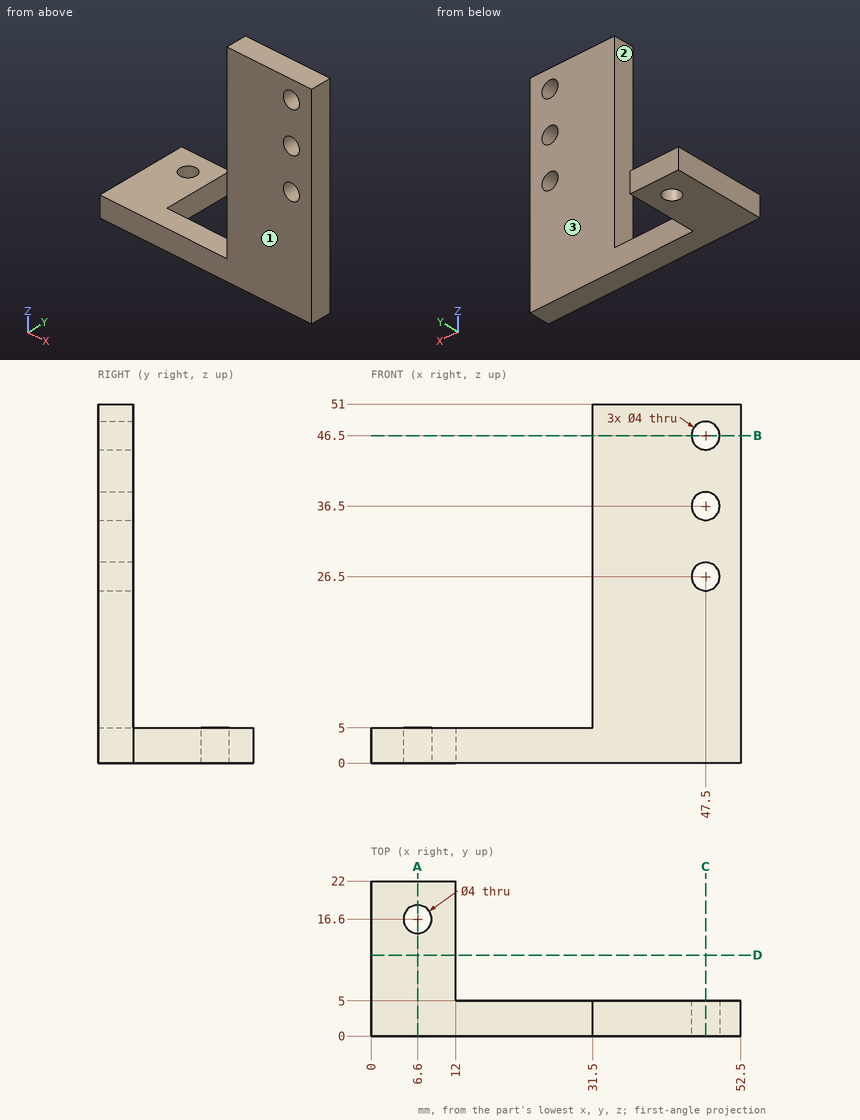
Design review of the part shown in the three views and the two pictorial views. Dimensions are in mm from the part's minimum x, y and z. A direction names the side the tool comes from. Give positions to 0.01 mm unless a question says otherwise; leave off trailing zeros. Loops run counter-clockwise (first coordinate to the right, second up) from the corner with the lowest first, then second, coordinate; pieces in that order, holes last. Notation, with made-up numbers: M -19,14 L 4,14 A19 ccw 4,50 Z; hole C 24,72 d7. An arc over 180 degrees is marked long. Put each result on its own line as item: value. Start each with the question number.
(1) Add section A-A, the plane x = 6.6. Write out the cut boundary in (y, z).
(2) Wall thickness on L1, parallel to X at y = 1.2, z = 46.5; L2, parallel to Y at x = 37.5, z = 25; L3, parallel to X at y = 2, z = 23: over which ranges is each line inside the solid? List them lowest first.
(3) Add section C-C, the plane x = 47.5. Write out the cut boundary in (y, z).
(4) Add section B-B, the plane z = 46.5. Write out the cut boundary in (x, y), then the cut area to 3 significant figures.
(5) Machinability: for the marked faces 1, 2 and 3, which of the approach directions +Z, -Z, +X, -X, +Y, -Y give a long, thin tool a straight path to every point of the face, cutting with its end or side? Answer none if there is none.
(6) For pin 1 (6.5 mm diameter, centred on x = 47.5, z = 36.5, fed in from +Y); pin 2 (2.5 mm diameter, centred on x = 6.6, y = 16.6, fed in from +Z); pin 3 (5.5 mm diameter, centred on y = 3, z = 32, fed in from -X); pin 4 (5.5 mm diameter, centred on y = 12, z = 3, fed in from +X), all flat-tipped, find the tip position at first contact; note any pin that passes through.
(7) Add section D-D, the plane y = 11.5. Write out the cut boundary in (x, z).
Result:
1. outline: M 0,0 L 14.6,0 L 14.6,5 L 0,5 Z; M 18.6,0 L 22,0 L 22,5 L 18.6,5 Z
2. L1: x = 31.5 to 45.5, 49.5 to 52.5
2. L2: y = 0 to 5
2. L3: x = 31.5 to 52.5
3. outline: M 0,0 L 5,0 L 5,24.5 L 0,24.5 Z; M 0,28.5 L 5,28.5 L 5,34.5 L 0,34.5 Z; M 0,38.5 L 5,38.5 L 5,44.5 L 0,44.5 Z; M 0,48.5 L 5,48.5 L 5,51 L 0,51 Z
4. outline: M 31.5,0 L 45.5,0 L 45.5,5 L 31.5,5 Z; M 49.5,0 L 52.5,0 L 52.5,5 L 49.5,5 Z
4. area: 85.0 mm^2
5. face 1: +Z, -Z, +X, -X, -Y
5. face 2: +Z, -X, +Y, -Y
5. face 3: +Z, -Z, +X, +Y
6. pin 1: stops at y = 5
6. pin 2: passes through
6. pin 3: stops at x = 31.5
6. pin 4: stops at x = 12
7. outline: M 0,0 L 12,0 L 12,5 L 0,5 Z
